from build123d import *

# Parameters (mm, degrees)
BOSS_EXTRUDE2_DEPTH = 40
CUT_EXTRUDE2_DEPTH  = 20
CUT_EXTRUDE3_START  = -20
CUT_EXTRUDE3_DEPTH  = 20
SKETCH9_R           = 15
CUT_EXTRUDE5_DEPTH  = 40
CUT_EXTRUDE6_DEPTH  = 20
SKETCH11_R          = 15
BOSS_EXTRUDE3_DEPTH = 80


with BuildPart() as part:
    # Sketch4 → Boss-Extrude2 (new, symmetric)
    with BuildSketch(Plane.XY):
        with BuildLine():
            Line((-250, 50), (250, 50))
            ThreePointArc((250, 50), (300, 0), (250, -50))
            Line((250, -50), (-250, -50))
            ThreePointArc((-250, -50), (-300, 0), (-250, 50))
        make_face()
    extrude(amount=BOSS_EXTRUDE2_DEPTH, both=True)

    # Sketch5 → Cut-Extrude2 (cut)
    with BuildSketch(Plane.XY.offset(40)):
        with BuildLine():
            Line((-150, 50), (-250, 50))
            ThreePointArc((-250, 50), (-300, 0), (-250, -50))
            Line((-250, -50), (-150, -50))
            ThreePointArc((-150, -50), (-200, 0), (-150, 50))
        make_face()
    extrude(amount=-CUT_EXTRUDE2_DEPTH, mode=Mode.SUBTRACT)

    # Sketch6 → Cut-Extrude3 (cut)
    with BuildSketch(Plane(origin=(0, 0, -40), x_dir=(-1, 0, 0), z_dir=(0, 0, -1)).offset(CUT_EXTRUDE3_START)):
        with BuildLine():
            Line((150, 50), (250, 50))
            ThreePointArc((250, 50), (300, 0), (250, -50))
            Line((250, -50), (150, -50))
            ThreePointArc((150, -50), (200, 0), (150, 50))
        make_face()
    extrude(amount=CUT_EXTRUDE3_DEPTH, mode=Mode.SUBTRACT)

    # Sketch9 → Cut-Extrude5 (cut)
    with BuildSketch(Plane.XY.offset(20)):
        with Locations((-250, 0)):
            Circle(SKETCH9_R)
    extrude(amount=-CUT_EXTRUDE5_DEPTH, mode=Mode.SUBTRACT)

    # Sketch10 → Cut-Extrude6 (cut, symmetric)
    with BuildSketch(Plane.XY):
        with BuildLine():
            Line((150, 50), (250, 50))
            ThreePointArc((250, 50), (300, 0), (250, -50))
            Line((250, -50), (150, -50))
            ThreePointArc((150, -50), (200, 0), (150, 50))
        make_face()
    extrude(amount=CUT_EXTRUDE6_DEPTH, both=True, mode=Mode.SUBTRACT)

    # Sketch11 → Boss-Extrude3 (add)
    with BuildSketch(Plane.XY.offset(40)):
        with Locations((250, 0)):
            Circle(SKETCH11_R)
    extrude(amount=-BOSS_EXTRUDE3_DEPTH)


solid = part.part
The listing builds one solid part. Answer for the finished solid, in the listing's coordinates (mm). A direction names the side the tool comes from. Round coordinates to 2 decimals unless told otherwise and drop trailing zeros. Order: outer loops, then holes, each group sorted by start corner. A loop starts at its lowest first (then second) coordinate and runs counter-clockwise, first axis right, second up. Notation, with made-up numbers: (5, -1.5) -> (64, -1.5) arc R32 cw to (64, 26.5) -> close; hole circle Ø10 at (-19.75, -26.5). An arc over 180 degrees is marked (long way). Put each result on its own line as item: value.
Q1. Each of these flat-tipped pins is pushed along its axis until it touches: P1, Ø10, axis at y = -25.5, z = -17.5, coming from the +X side; P2, Ø6, axis at y = -7, z = -28, coming from the +X side. Where does it stop, or does it pass through?
Results list:
P1: x = 295.3
P2: x = 299.84
Q2. Section D-D, the plane z = -29 is taken. Write down the section's boundary in (x, y).
Results list:
outline: (-150, -50) -> (250, -50) arc R50 ccw to (250, 50) -> (-150, 50) arc R50 ccw to start
Q3. Determine the mould class of faces 1 (the cylindrical face through (299.988, 1.099, -29.86)), 2 (the flat face through (53, 1, -40)), 3 (the cylindrical face through (263.856, -5.745, 0.28)) for opening direction X: pulls with the +X half, pulls with the -X half, needs draft (parallel to the pull), parting line crosses it, or undercut.
Results list:
face 1: pulls with the +X half
face 2: needs draft
face 3: undercut
Q4. Which of the six approach directions +Z, -Z, +X, -X, +Y, -Y give full straight-line access (tool end or side, diameter ignored) to faces 4 (the cylindrical face through (-199.988, -1.099, 30.14)), 5 (the flat face through (226, 1, -20)), 6 (the cylindrical face through (-199.988, -1.099, -29.86))?
Results list:
face 4: +Z, -X
face 5: none
face 6: -Z, -X
Q5. Consider line 1 along Y through (x, z) = (-250, -7); line 2 along Z through (x, y) = (-203.5, 45.5); line 3 along Z through (x, y) = (254, -26). Determine where each line is inside the solid, lowest interval first.
Results list:
line 1: -50 to -15, 15 to 50
line 2: -20 to 20
line 3: -40 to -20, 20 to 40
Q6. Section C-C, the plane y = -40 is taken. Write down the section's boundary in (x, z).
Results list:
outline: (-280, -20) -> (-180, -20) -> (-180, -40) -> (280, -40) -> (280, -20) -> (180, -20) -> (180, 20) -> (280, 20) -> (280, 40) -> (-180, 40) -> (-180, 20) -> (-280, 20) -> close
Q7. Section B-B, the plane z = 0.5 is taken. Write down the section's boundary in (x, y).
Results list:
outline: (-250, -50) -> (150, -50) arc R50 ccw to (150, 50) -> (-250, 50) arc R50 ccw to start; circle Ø30 at (250, 0); hole circle Ø30 at (-250, 0)
Q8. Section A-A, the plane y = 0 is taken. Write down the section's boundary in (x, z), and give its area (3 significant figures).
Results list:
outline: (-300, -20) -> (-265, -20) -> (-265, 20) -> (-300, 20) -> close; (-235, -20) -> (-200, -20) -> (-200, -40) -> (300, -40) -> (300, -20) -> (265, -20) -> (265, 20) -> (300, 20) -> (300, 40) -> (-200, 40) -> (-200, 20) -> (-235, 20) -> close; hole (200, -20) -> (235, -20) -> (235, 20) -> (200, 20) -> close
area: 40,000 mm^2
